Design review of the part shown in the three views and the two pictorial views. Dimensions are in mm from the part's minimum x, y and z. A direction names the side the tool comes from. Coordinates: 2 decimals unless noted, no trailing zeros. Loops run counter-clockwise (first coordinate to the right, second up) from the corner with the lowest first, then second, coordinate; pieces in that order, holes last. Notation, with made-up numbers: M -31.75,-36.75 L 2.25,-36.75 A30 cw 2.25,-13.75 Z; hole C 24.5,43.5 d5. An arc over 180 degrees is marked long. Put each result on its own line as item: value. Start each with the question number.
(1) The part is to be moulded in two halves that separate along X. For the marked faces 1, 2 and 3, say which applies: +X half, -X half, draft (parallel to the pull), parting line (faces both ways), or undercut.
(2) Take a section at A-A, the plane z = 61.5. Give the boundary of the cut face in (x, y), then the cut area to 3 significant figures.
(3) For the marked faces 4 and 5, list the 3-axis set-ups (+Z, -Z, +X, -X, +Y, -Y) from which the entire face can be reached by the end or side of a thin tool; tool diameter is ignored.
(4) Clearance check with flat-ended pins moving along their axes: pin 1 (12 mm diameter, centred on x = 112.5, y = 6.5, fed in from +Z); pin 2 (20 mm diameter, centred on x = 75.5, z = 73.5, fed in from -Y); pin 3 (10 mm diameter, centred on y = 21.5, z = 89.5, fed in from +X). State where each tip first meets the part, or that it passes through.
(5) Take a section at C-C, the plane y = 18. Give the boundary of the cut face in (x, z).
(6) For probe 1 along Y at (x, z) = (37, 22); probe 2 along Y at (x, z) = (61.5, 59); probe 3 along X at (y, z) = (23.25, 35), list the stretches that pass through material, from the lowest coordinate up. Write a range as [from, to].
(7) Take a section at D-D, the plane z = 43. Give the boundary of the cut face in (x, y), then the cut area to 3 significant figures.
(8) Take a section at B-B, the plane x = 65. Give the boundary of the cut face in (y, z).
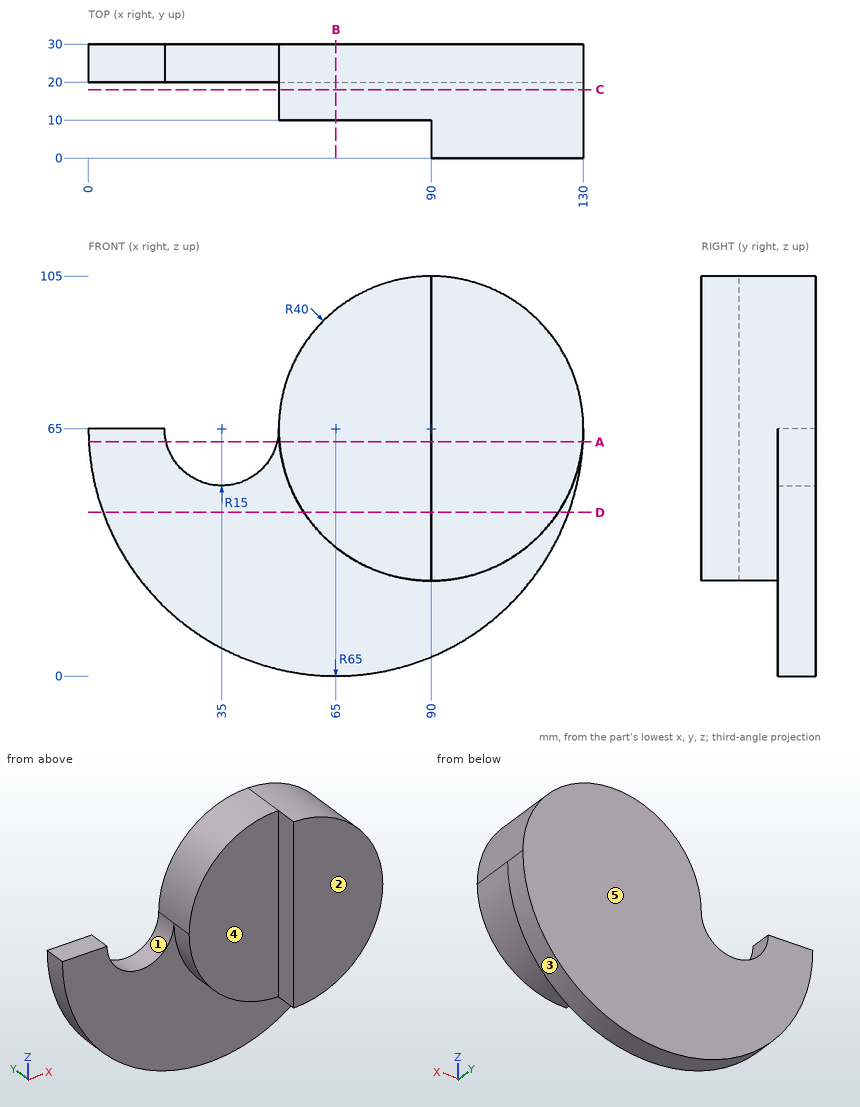
Computed values:
1. face 1: undercut
1. face 2: draft
1. face 3: parting line
2. outline: M 0.09,20 L 20.41,20 L 20.41,30 L 0.09,30 Z; M 49.59,20 L 50.15,20 L 50.15,10 L 90,10 L 90,0 L 129.85,0 L 129.85,20 L 129.91,20 L 129.91,30 L 49.59,30 Z
2. area: 2,200 mm^2
3. face 4: +Z, -Z, -X, -Y
3. face 5: +Z, -Z, +X, -X, +Y
4. pin 1: stops at z = 101.44
4. pin 2: stops at y = 10
4. pin 3: stops at x = 124.92
5. outline: M 50,65 A40 ccw 90,25 A40 ccw 130,65 A40 ccw 90,105 A40 ccw Z
6. probe 1: y = [20, 30]
6. probe 2: y = [10, 30]
6. probe 3: x = [7.34, 122.66]
7. outline: M 3.84,20 L 56.59,20 L 56.59,10 L 90,10 L 90,0 L 123.41,0 L 123.41,20 L 126.16,20 L 126.16,30 L 3.84,30 Z
7. area: 2,230 mm^2
8. outline: M 10,33.78 L 20,33.78 L 20,0 L 30,0 L 30,96.22 L 10,96.22 Z
